Autodesk Inventor part; units mm, degrees
ref_plane "YZ Plane" through (0, 0, 0) normal (1, 0, 0) x (0, 1, 0)
ref_plane "XZ Plane" through (0, 0, 0) normal (0, 1, 0) x (-1, 0, 0)
ref_plane "XY Plane" through (0, 0, 0) normal (0, 0, 1) x (1, 0, 0)
sketch "Sketch1" plane through (0, 0, 0) normal (0, 1, 0) x (-1, 0, 0)
  line L0 (100, 100) -> (100, -100)
  line L1 (100, -100) -> (-100, -100)
  line L2 (-100, -100) -> (-100, 100)
  line L3 (-100, 100) -> (100, 100)
  line L4 (100, 100) -> (-100, -100) construction
  line L5 (100, -100) -> (-100, 100) construction
  point P0 (0, 0)
  dimension "d0" = 200
  dimension "d1" = 200
extrude "Extrusion1" add sketch "Sketch1" along normal blind 3
sketch "Sketch3" plane through (0, 3, 0) normal (0, 1, 0) x (1, 0, 0)
  line L0 (100, -100) -> (100, 100)
  line L1 (100, 100) -> (100, -100)
  line L2 (100, -100) -> (97, -100)
  line L3 (97, -100) -> (97, 100)
  line L4 (97, 100) -> (100, 100)
  dimension "d4" = 3
extrude "Extrusion2" add sketch "Sketch3" along normal blind 197
sketch "Sketch4" plane through (0, 3, 0) normal (0, 1, 0) x (1, 0, 0)
  line L0 (-100, 100) -> (97, 100)
  line L1 (97, 100) -> (97, 97)
  line L2 (97, 97) -> (-100, 97)
  line L3 (-100, 97) -> (-100, 100)
  dimension "d7" = 3
extrude "Extrusion3" add sketch "Sketch4" along normal blind 197
properties part number "Chassis Constraints"
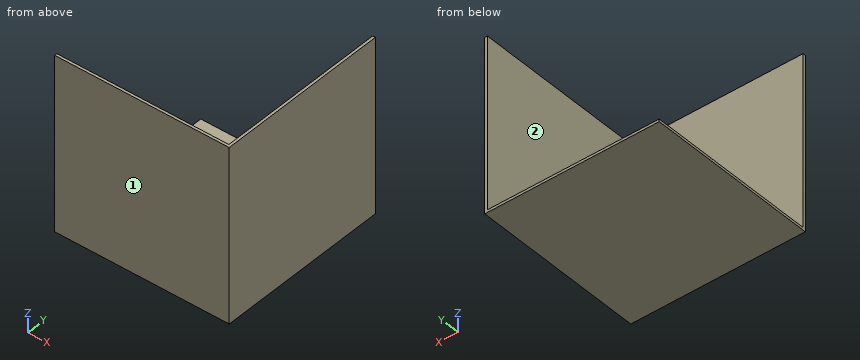
For this review, take the finished solid that the model builds, in its own axes (mm). Face numbers are marked on the shaded views. A direction names the side the tool comes from. Round coordinates to 2 decimals unless told otherwise and drop trailing zeros. Loops run counter-clockwise (first coordinate to the right, second up) from the corner with the lowest first, then second, coordinate; pieces in that order, holes last.
(1) We need section A-A (x = 13). Give the boundary of the cut face in (y, z).
Returned:
outline: (0, -100) - (200, -100) - (200, -97) - (3, -97) - (3, 100) - (0, 100) - close
(2) We need section B-B (y = 53). Give the boundary of the cut face in (x, z), plus the area to 3 significant figures.
Returned:
outline: (-100, -100) - (100, -100) - (100, 100) - (97, 100) - (97, -97) - (-100, -97) - close
area: 1,190 mm2
(3) Wall thickness on line 1 along X through (y, z) = (177.5, -78); line 2 along Y through (x, z) = (-23, 81); line 3 along Z through (x, y) = (-3.5, 94): over which ranges is each line inside the solid? List them lowest first.
Returned:
line 1: x = 97 to 100
line 2: y = 0 to 3
line 3: z = -100 to -97
(4) Clearance check with flat-ended pins moving along their axes: P1, Ø3, axis at x = 47.5, y = 38, coming from the +Z side; P2, Ø3, axis at y = 52.5, z = 45, coming from the -X side; P3, Ø12, axis at x = -9.5, z = 15.5, coming from the +Y side. State where each tip first meets the part, or that it passes through.
Returned:
P1: stops at z = -97
P2: stops at x = 97
P3: stops at y = 3
(5) Tool access review of the marked faces 1 and 2: name each direction out of +Z, -Z, +X, -X, +Y, -Y from which nothing blocks a thin tool from reaching the whole face with its end or side.
Returned:
face 1: +Z, -Z, +X, -X, -Y
face 2: +Z, -X, +Y
